Here's how the part is built. I have some questions about the finished solid (model axes, mm). Face numbers are marked on the shaded views. A direction names the side the tool comes from. Coordinates: 2 decimals unless noted, no trailing zeros. Write each loop counter-clockwise with the first axis right and the second up, starting at its lowest first coordinate (ties: lowest second). Pieces come first, ordered by that corner, then holes.
(1) Thinking about a two-plate mould opening in Z: for the marked faces 4, 5 and 6, which applies, released by +Z, released by -Z, zero draft, split by the parting line, or undercut?
(2) Imagine slicing it at A-A, the plane z = 26. List the corners of the cut face in (x, y) for me (3 decimals), plus the area to 3 significant figures.
(3) Imagine slicing it at D-D, the plane z = -5.5. List the corners of the cut face in (x, y) for me (3 decimals).
(4) For pin 1 Ø6 at (x, y) = (15.5, 40.5) entering from +Z; pin 2 Ø6 at (y, z) = (-15, 33) entering from +X; pin 3 Ø5.5 at (x, y) = (-36.37, 7.54) entering from -Z; pin 4 Ø13.5 at (x, y) = (-7, 6) entering from -Z, each with a flat end and sliding along its axis, tell me the tip position at first contact or that it passes through.
(5) Which directions (+Z, -Z, +X, -X, +Y, -Y) give clear straight access to the entire face, cutting with the end or side of a thin tool? Please do the marked faces 1, 2 and 3.
(6) Imagine slicing it at B-B, the plane x = 0. State how many separate pieces and enclosed holes the cut face has, plus the area to 3 significant figures.
(7) Please list where these lines run through material, in increasing order: probe 1 along X at (y, z) = (0.5, 25.5); probe 2 along Z at (x, y) = (-4.5, -31.5) (3 decimals); probe 3 along Z at (x, y) = (-33, 41).
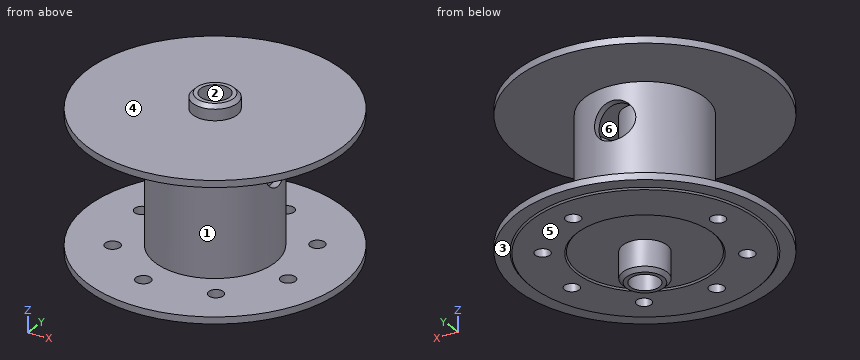
Autodesk Inventor part; units mm, degrees
ref_plane "Work Plane1" through (25.6794, 0, 2.921) normal (1, 0, 0) x (0, 1, 0)
ref_plane "XZ Plane" through (0, 0, 0) normal (0, 1, 0) x (-1, 0, 0)
ref_plane "XY Plane" through (0, 0, 0) normal (0, 0, 1) x (1, 0, 0)
sketch "Sketch1" plane through (0, 0, 0) normal (0, 0, 1) x (1, 0, 0)
  circle A0 centre (0, 0) radius 54.8005
  dimension "d0" = 109.601
extrude "Extrusion1" add sketch "Sketch1" along normal blind 2.921
sketch "Sketch2" plane through (0, 0, 2.921) normal (0, 0, 1) x (1, 0, 0)
  circle A0 centre (0, 0) radius 54.8005
  circle A1 centre (0, 0) radius 25.6794
  circle A2 centre (0, 0) radius 22.7584
  dimension "d3" = 51.3588
  dimension "d17" = 2.921
extrude "Extrusion2" add sketch "Sketch2" along normal blind 53.467 contours A1
sketch "Sketch3" plane through (0, 0, 56.388) normal (0, 0, 1) x (1, 0, 0)
  circle A0 centre (0, 0) radius 25.6794
  circle A1 centre (0, 0) radius 54.8005
  circle A2 centre (0, 0) radius 54.8005
extrude "Extrusion3" add sketch "Sketch3" along normal blind 2.921 contours A0 | A1
sketch "Sketch4" plane through (0, 0, 59.309) normal (0, 0, 1) x (1, 0, 0)
  circle A0 centre (0, 0) radius 54.8005
  circle A1 centre (0, 0) radius 9.525
  dimension "d8" = 19.05
extrude "Extrusion4" add sketch "Sketch4" along normal blind 6.35 contours A1
sketch "Sketch5" plane through (0, 0, 65.659) normal (0, 0, 1) x (1, 0, 0)
  circle A0 centre (0, 0) radius 9.525
  circle A1 centre (0, 0) radius 6.223
  dimension "d11" = 12.446
sketch "Sketch6" plane through (0, 0, 0) normal (0, 0, -1) x (-1, 0, 0)
  circle A0 centre (0, 0) radius 9.525
  circle A1 centre (0, 0) radius 9.525
  circle A2 centre (0, 0) radius 9.525
  dimension "d12" = 19.05
extrude "Extrusion5" add sketch "Sketch6" along normal blind 12.7
extrude "Extrusion6" cut sketch "Sketch5" against normal through all contours A1
sketch "Sketch7" plane through (0, 0, 2.921) normal (0, 0, 1) x (1, 0, 0)
  circle A0 centre (0, 0) radius 6.223
  circle A1 centre (0, 0) radius 6.223
  circle A2 centre (0, 0) radius 9.525
extrude "Extrusion7" add sketch "Sketch7" along normal through all
chamfer "Chamfer1" distance 1.5875 angle 45 2 edges at (-9.525, 0, 65.659) (9.525, 0, -12.7)
ref_plane "Work Plane1" through (25.6794, 0, 2.921) normal (1, 0, 0) x (0, 1, 0)
sketch "Sketch8" plane through (25.6794, 0, 2.921) normal (1, 0, 0) x (0, 1, 0)
  line L0 (-54.8005, 53.467) -> (54.8005, 53.467)
  line L1 (-25.6794, 53.467) -> (25.6794, 53.467)
  line L2 (-54.8005, 0) -> (54.8005, 0)
  line L3 (-25.6794, 0) -> (25.6794, 0)
  circle A0 centre (2.6963, 38.862) radius 8.2931
  point P0 (0, -2.921)
  dimension "d23" = 14.605
  dimension "d24" = 16.5862
extrude "Extrusion8" cut sketch "Sketch8" against normal blind 12.7
pattern_circular "Circular Pattern1" count 2 over 90 about axis through (0, 0, 2.921) along (0, 0, 1) of "Extrusion8"
sketch "Sketch9" plane through (0, 0, 0) normal (0, 0, -1) x (-1, 0, 0)
  circle A0 centre (0, 0) radius 54.8005
  circle A1 centre (0, 0) radius 28.5115
  circle A2 centre (0, 0) radius 48.9585
  dimension "d30" = 57.023
  dimension "d31" = 97.917
extrude "Extrusion9" add sketch "Sketch9" along normal blind 0.635 contours A2
chamfer "Chamfer2" distance 0.635 angle 45 2 edges at (48.9585, 0, -0.635) (28.5115, 0, -0.635)
sketch "Sketch12" plane through (0, 0, 2.921) normal (0, 0, 1) x (1, 0, 0)
  circle A0 centre (0, 0) radius 28.5115
  circle A1 centre (31.0504, 20.3913) radius 3.175
  circle A2 centre (-31.0504, -20.3913) radius 3.175
  circle A3 centre (20.3913, -31.0504) radius 3.175
  circle A4 centre (-36.3748, 7.5371) radius 3.175
  circle A5 centre (7.5371, 36.3748) radius 3.175
  circle A6 centre (36.3748, -7.5371) radius 3.175
  circle A7 centre (-7.5371, -36.3748) radius 3.175
  arc A8 (19.7771, 37.7111) -> (20.5429, 44.5183) centre (-8.1746, 44.3026) ccw
  arc A9 (21.6617, 36.661) -> (19.7771, 37.7111) centre (0, 0) ccw
  arc A10 (27.0474, 40.8941) -> (21.6617, 36.661) centre (41.9748, 16.3602) ccw
  arc A11 (29.0839, 39.4717) -> (27.0474, 40.8941) centre (0, 0) ccw
  arc A12 (26.9634, 32.958) -> (29.0839, 39.4717) centre (0.9108, 45.0412) ccw
  arc A13 (28.5981, 31.55) -> (26.9634, 32.958) centre (0, 0) ccw
  arc A14 (34.7256, 34.6124) -> (28.5981, 31.55) centre (44.4089, 7.5758) ccw
  arc A15 (36.4341, 32.8092) -> (34.7256, 34.6124) centre (0, 0) ccw
  arc A16 (33.0459, 26.8557) -> (36.4341, 32.8092) centre (9.9589, 43.9359) ccw
  arc A17 (34.3637, 25.1474) -> (33.0459, 26.8557) centre (0, 0) ccw
  arc A18 (40.9822, 26.9137) -> (34.3637, 25.1474) centre (45.0248, -1.5187) ccw
  arc A19 (42.2928, 24.8034) -> (40.9822, 26.9137) centre (0, 0) ccw
  arc A20 (37.7754, 19.6538) -> (42.2928, 24.8034) centre (18.5992, 41.0318) ccw
  arc A21 (38.7224, 17.7153) -> (37.7754, 19.6538) centre (0, 0) ccw
  arc A22 (45.561, 18.1131) -> (38.7224, 17.7153) centre (43.7975, -10.551) ccw
  arc A23 (46.4199, 15.7822) -> (45.561, 18.1131) centre (0, 0) ccw
  arc A24 (40.9585, 11.6474) -> (46.4199, 15.7822) centre (26.4782, 36.4479) ccw
  arc A25 (41.4958, 9.5579) -> (40.9585, 11.6474) centre (0, 0) ccw
  arc A26 (48.2745, 8.571) -> (41.4958, 9.5579) centre (40.777, -19.1514) ccw
  arc A27 (48.6467, 6.1149) -> (48.2745, 8.571) centre (0, 0) ccw
  arc A28 (42.4646, 3.1641) -> (48.6467, 6.1149) centre (33.2731, 30.3718) ccw
  arc A29 (42.5704, 1.0092) -> (42.4646, 3.1641) centre (0, 0) ccw
  arc A30 (49.0116, -1.3221) -> (42.5704, 1.0092) centre (36.0871, -26.9677) ccw
  arc A31 (48.8818, -3.8028) -> (49.0116, -1.3221) centre (0, 0) ccw
  arc A32 (42.2323, -5.4487) -> (48.8818, -3.8028) centre (38.7058, 23.0522) ccw
  arc A33 (41.9021, -7.5808) -> (42.2323, -5.4487) centre (0, 0) ccw
  arc A34 (47.7422, -11.161) -> (41.9021, -7.5808) centre (29.9199, -33.68) ccw
  arc A35 (47.1157, -13.5648) -> (47.7422, -11.161) centre (0, 0) ccw
  arc A36 (40.271, -13.8385) -> (47.1157, -13.5648) centre (42.5538, 14.789) ccw
  arc A37 (39.5184, -15.8604) -> (40.271, -13.8385) centre (0, 0) ccw
  arc A38 (44.5183, -20.543) -> (39.5184, -15.8604) centre (22.5277, -39.0134) ccw
  arc A39 (43.4206, -22.7714) -> (44.5183, -20.543) centre (0, 0) ccw
  arc A40 (36.661, -21.6617) -> (43.4206, -22.7714) centre (44.6597, 5.9202) ccw
  arc A41 (35.5168, -23.4908) -> (36.661, -21.6617) centre (0, 0) ccw
  arc A42 (39.4717, -29.0839) -> (35.5168, -23.4908) centre (14.2132, -42.7496) ccw
  arc A43 (37.948, -31.0458) -> (39.4717, -29.0839) centre (0, 0) ccw
  arc A44 (31.55, -28.5981) -> (37.948, -31.0458) centre (44.9373, -3.1909) ccw
  arc A45 (30.0611, -30.1594) -> (31.55, -28.5981) centre (0, 0) ccw
  arc A46 (32.8092, -36.4341) -> (30.0611, -30.1594) centre (5.3168, -44.7356) ccw
  arc A47 (30.9217, -38.0491) -> (32.8092, -36.4341) centre (0, 0) ccw
  arc A48 (25.1475, -34.3637) -> (30.9217, -38.0491) centre (43.3751, -12.1714) ccw
  arc A49 (23.3747, -35.5933) -> (25.1475, -34.3637) centre (0, 0) ccw
  arc A50 (24.8034, -42.2928) -> (23.3747, -35.5933) centre (-3.7972, -44.8901) ccw
  arc A51 (22.6295, -43.4948) -> (24.8034, -42.2928) centre (0, 0) ccw
  arc A52 (17.7153, -38.7224) -> (22.6295, -43.4948) centre (40.0371, -20.6536) ccw
  arc A53 (15.7313, -39.57) -> (17.7153, -38.7224) centre (0, 0) ccw
  arc A54 (15.7822, -46.4199) -> (15.7313, -39.57) centre (-12.7558, -43.2068) ccw
  arc A55 (13.4108, -47.1597) -> (15.7822, -46.4199) centre (0, 0) ccw
  arc A56 (9.5579, -41.4958) -> (13.4108, -47.1597) centre (35.06, -28.2902) ccw
  arc A57 (7.4439, -41.9267) -> (9.5579, -41.4958) centre (0, 0) ccw
  arc A58 (6.1149, -48.6467) -> (7.4439, -41.9267) centre (-21.1922, -39.7547) ccw
  arc A59 (3.6431, -48.8939) -> (6.1149, -48.6467) centre (0, 0) ccw
  arc A60 (1.0092, -42.5704) -> (3.6431, -48.8939) centre (28.6475, -34.7687) ccw
  arc A61 (-1.1482, -42.5669) -> (1.0092, -42.5704) centre (0, 0) ccw
  arc A62 (-3.8028, -48.8818) -> (-1.1482, -42.5669) centre (-28.7609, -34.6749) ccw
  arc A63 (-6.2737, -48.6264) -> (-3.8028, -48.8818) centre (0, 0) ccw
  arc A64 (-7.5808, -41.9021) -> (-6.2737, -48.6264) centre (21.0622, -39.8237) ccw
  arc A65 (-9.6934, -41.4644) -> (-7.5808, -41.9021) centre (0, 0) ccw
  arc A66 (-13.5648, -47.1157) -> (-9.6934, -41.4644) centre (-35.1522, -28.1756) ccw
  arc A67 (-15.9337, -46.3682) -> (-13.5648, -47.1157) centre (0, 0) ccw
  arc A68 (-15.8604, -39.5184) -> (-15.9337, -46.3682) centre (12.6147, -43.2483) ccw
  arc A69 (-17.8417, -38.6644) -> (-15.8604, -39.5184) centre (0, 0) ccw
  arc A70 (-22.7714, -43.4207) -> (-17.8417, -38.6644) centre (-40.1043, -20.5228) ccw
  arc A71 (-24.9414, -42.2116) -> (-22.7714, -43.4207) centre (0, 0) ccw
  arc A72 (-23.4908, -35.5168) -> (-24.9414, -42.2116) centre (3.6506, -44.9023) ccw
  arc A73 (-25.2595, -34.2814) -> (-23.4908, -35.5168) centre (0, 0) ccw
  arc A74 (-31.0458, -37.948) -> (-25.2595, -34.2814) centre (-43.4146, -12.0297) ccw
  arc A75 (-32.928, -36.3268) -> (-31.0458, -37.948) centre (0, 0) ccw
  arc A76 (-30.1594, -30.0611) -> (-32.928, -36.3268) centre (-5.4629, -44.718) ccw
  arc A77 (-31.6432, -28.4949) -> (-30.1594, -30.0611) centre (0, 0) ccw
  arc A78 (-38.0491, -30.9217) -> (-31.6432, -28.4949) centre (-44.9475, -3.0442) ccw
  arc A79 (-39.5665, -28.9549) -> (-38.0491, -30.9217) centre (0, 0) ccw
  arc A80 (-35.5933, -23.3747) -> (-39.5665, -28.9549) centre (-14.3527, -42.7029) ccw
  arc A81 (-36.7315, -21.5419) -> (-35.5933, -23.3747) centre (0, 0) ccw
  arc A82 (-43.4948, -22.6295) -> (-36.7315, -21.5419) centre (-44.6402, 6.066) ccw
  arc A83 (-44.5851, -20.3975) -> (-43.4948, -22.6295) centre (0, 0) ccw
  arc A84 (-39.57, -15.7313) -> (-44.5851, -20.3975) centre (-22.6549, -38.9396) ccw
  arc A85 (-40.316, -13.707) -> (-39.57, -15.7313) centre (0, 0) ccw
  arc A86 (-47.1597, -13.4108) -> (-40.316, -13.707) centre (-42.5053, 14.9278) ccw
  arc A87 (-47.7784, -11.005) -> (-47.1597, -13.4108) centre (0, 0) ccw
  arc A88 (-41.9267, -7.4439) -> (-47.7784, -11.005) centre (-30.0297, -33.5821) ccw
  arc A89 (-42.2499, -5.3108) -> (-41.9267, -7.4439) centre (0, 0) ccw
  arc A90 (-48.8939, -3.6431) -> (-42.2499, -5.3108) centre (-38.6303, 23.1785) ccw
  arc A91 (-49.0157, -1.162) -> (-48.8939, -3.6431) centre (0, 0) ccw
  arc A92 (-42.5669, 1.1482) -> (-49.0157, -1.162) centre (-36.175, -26.8498) ccw
  arc A93 (-42.4541, 3.3027) -> (-42.5669, 1.1482) centre (0, 0) ccw
  arc A94 (-48.6264, 6.2737) -> (-42.4541, 3.3027) centre (-33.1737, 30.4803) ccw
  arc A95 (-48.2463, 8.7285) -> (-48.6264, 6.2737) centre (0, 0) ccw
  arc A96 (-41.4644, 9.6934) -> (-48.2463, 8.7285) centre (-40.8393, -19.0182) ccw
  arc A97 (-40.9202, 11.7811) -> (-41.4644, 9.6934) centre (0, 0) ccw
  arc A98 (-46.3682, 15.9337) -> (-40.9202, 11.7811) centre (-26.359, 36.5341) ccw
  arc A99 (-45.5016, 18.2618) -> (-46.3682, 15.9337) centre (0, 0) ccw
  arc A100 (-38.6644, 17.8417) -> (-45.5016, 18.2618) centre (-43.8317, -10.408) ccw
  arc A101 (-37.7111, 19.7771) -> (-38.6644, 17.8417) centre (0, 0) ccw
  arc A102 (-42.2116, 24.9414) -> (-37.7111, 19.7771) centre (-18.4652, 41.0923) ccw
  arc A103 (-40.8941, 27.0474) -> (-42.2116, 24.9414) centre (0, 0) ccw
  arc A104 (-34.2814, 25.2595) -> (-40.8941, 27.0474) centre (-45.0295, -1.3717) ccw
  arc A105 (-32.958, 26.9634) -> (-34.2814, 25.2595) centre (0, 0) ccw
  arc A106 (-36.3268, 32.928) -> (-32.958, 26.9634) centre (-9.8154, 43.9682) ccw
  arc A107 (-34.6124, 34.7256) -> (-36.3268, 32.928) centre (0, 0) ccw
  arc A108 (-28.4949, 31.6432) -> (-34.6124, 34.7256) centre (-44.3839, 7.7208) ccw
  arc A109 (-26.8557, 33.0459) -> (-28.4949, 31.6432) centre (0, 0) ccw
  arc A110 (-28.9549, 39.5665) -> (-26.8557, 33.0459) centre (-0.7637, 45.044) ccw
  arc A111 (-26.9137, 40.9822) -> (-28.9549, 39.5665) centre (0, 0) ccw
  arc A112 (-21.5419, 36.7315) -> (-26.9137, 40.9822) centre (-41.9212, 16.4971) ccw
  arc A113 (-19.6538, 37.7754) -> (-21.5419, 36.7315) centre (0, 0) ccw
  arc A114 (-20.3975, 44.5851) -> (-19.6538, 37.7754) centre (8.3192, 44.2756) ccw
  arc A115 (-18.1131, 45.561) -> (-20.3975, 44.5851) centre (0, 0) ccw
  arc A116 (-13.707, 40.316) -> (-18.1131, 45.561) centre (-37.7422, 24.5981) ccw
  arc A117 (-11.6474, 40.9585) -> (-13.707, 40.316) centre (0, 0) ccw
  arc A118 (-11.005, 47.7784) -> (-11.6474, 40.9585) centre (17.0615, 41.6947) ccw
  arc A119 (-8.571, 48.2745) -> (-11.005, 47.7784) centre (0, 0) ccw
  arc A120 (-5.3108, 42.2499) -> (-8.571, 48.2745) centre (-32.018, 31.692) ccw
  arc A121 (-3.1641, 42.4646) -> (-5.3108, 42.2499) centre (0, 0) ccw
  arc A122 (-1.162, 49.0157) -> (-3.1641, 42.4646) centre (25.1053, 37.4067) ccw
  arc A123 (1.3221, 49.0116) -> (-1.162, 49.0157) centre (0, 0) ccw
  arc A124 (3.3027, 42.4541) -> (1.3221, 49.0116) centre (-24.9831, 37.4885) ccw
  arc A125 (5.4487, 42.2323) -> (3.3027, 42.4541) centre (0, 0) ccw
  arc A126 (8.7285, 48.2463) -> (5.4487, 42.2323) centre (32.1214, 31.5873) ccw
  arc A127 (11.161, 47.7422) -> (8.7285, 48.2463) centre (0, 0) ccw
  arc A128 (11.7811, 40.9202) -> (11.161, 47.7422) centre (-16.9253, 41.7502) ccw
  arc A129 (13.8385, 40.271) -> (11.7811, 40.9202) centre (0, 0) ccw
  arc A130 (18.2618, 45.5016) -> (13.8385, 40.271) centre (37.8223, 24.4748) ccw
  arc A131 (20.5429, 44.5183) -> (18.2618, 45.5016) centre (0, 0) ccw
extrude "Extrusion11" cut sketch "Sketch12" against normal blind 25.4 contours A1 | A2 | A3 | A4 | A5 | A6 | A7
properties part number "Spool 1764"
Recorded:
1. face 4: released by +Z
1. face 5: released by -Z
1. face 6: undercut
2. outline: circle Ø51.359 at (0, 0); circle Ø19.05 at (0, 0); hole circle Ø45.517 at (0, 0); hole circle Ø12.446 at (0, 0)
2. area: 608 mm2
3. outline: circle Ø19.05 at (0, 0); hole circle Ø12.446 at (0, 0)
4. pin 1: stops at z = 59.31
4. pin 2: stops at x = 22.7
4. pin 3: stops at z = 56.39
4. pin 4: stops at z = -12.7
5. face 1: none
5. face 2: +Z, -Z
5. face 3: -Z
6. separate pieces: 2
6. enclosed holes: 1
6. area: 1,330 mm2
7. probe 1: x = -25.67 to -22.75, -9.51 to -6.2, 6.2 to 9.51, 22.75 to 25.67
7. probe 2: z = -0.635 to 2.921, 56.388 to 59.309
7. probe 3: z = 0 to 2.92, 56.39 to 59.31
